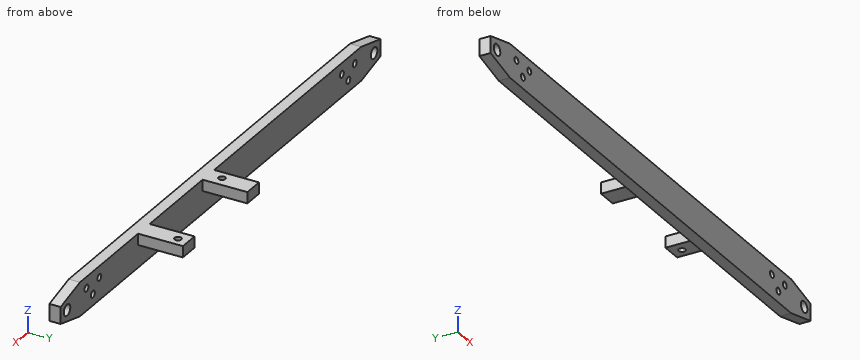
from build123d import *

# Parameters (mm, degrees)
BOSS_EXTRUDE1_DEPTH = 5
SKETCH2_R           = 1.5
SKETCH2_R_2         = 2.5
CUT_EXTRUDE1_DEPTH  = 5
SKETCH4_W           = 9
SKETCH4_H           = 5
BOSS_EXTRUDE2_DEPTH = 20
SKETCH6_R           = 1.5
CUT_EXTRUDE2_DEPTH  = 5


with BuildPart() as part:
    # Sketch1 → Boss-Extrude1 (new body)
    with BuildSketch(Plane(origin=(0, 0, 0), x_dir=(1, 0, 0), z_dir=(0, 1, 0))):
        Polygon((-67.598283163, 7.319100723), (-52.598283163, 3.569100723), (165.401716837, 3.569100723), (180.401716837, 7.319100723), (180.401716837, 14.819100723), (165.401716837, 18.569100723), (-52.598283163, 18.569100723), (-67.598283163, 14.819100723), align=None)
    extrude(amount=BOSS_EXTRUDE1_DEPTH)

    # Sketch2 → Cut-Extrude1 (cut)
    with BuildSketch(Plane(origin=(0, 5, 0), x_dir=(1, 0, 0), z_dir=(0, 1, 0))):
        with Locations(Location((155.401716837, 13.569100723, 0), (0, 0, 270))):
            Circle(SKETCH2_R)
        with Locations(Location((160.401716837, 8.569100723, 0), (0, 0, 270))):
            Circle(SKETCH2_R)
        with Locations(Location((150.401716837, 8.569100723, 0), (0, 0, 270))):
            Circle(SKETCH2_R)
        with Locations(Location((-47.598283163, 8.569100723, 0), (0, 0, 270))):
            Circle(SKETCH2_R)
        with Locations(Location((-37.598283163, 8.569100723, 0), (0, 0, 270))):
            Circle(SKETCH2_R)
        with Locations(Location((-42.598283163, 13.569100723, 0), (0, 0, 270))):
            Circle(SKETCH2_R)
        with Locations(Location((-62.598283163, 11.069100723, 0), (0, 0, 270))):
            Circle(SKETCH2_R_2)
        with Locations(Location((175.401716837, 11.069100723, 0), (0, 0, 270))):
            Circle(SKETCH2_R_2)
    extrude(amount=-CUT_EXTRUDE1_DEPTH, mode=Mode.SUBTRACT)

    # Sketch4 → Boss-Extrude2 (add)
    with BuildSketch(Plane(origin=(-36.696088283, 5, 1.62747237), x_dir=(1, 0, 0), z_dir=(0, 1, 0))):
        with Locations((102.59780512, 7.696573093)):
            Rectangle(SKETCH4_W, SKETCH4_H)
        with Locations((152.59780512, 7.696573093)):
            Rectangle(SKETCH4_W, SKETCH4_H)
    extrude(amount=BOSS_EXTRUDE2_DEPTH)

    # Sketch6 → Cut-Extrude2 (cut)
    with BuildSketch(Plane(origin=(-36.696088283, 0, -3.569100723), x_dir=(1, 0, 0), z_dir=(0, 0, 1))):
        with Locations((102.29780512, 10.9)):
            Circle(SKETCH6_R)
        with Locations((152.89780512, 20.4)):
            Circle(SKETCH6_R)
    extrude(amount=-CUT_EXTRUDE2_DEPTH, mode=Mode.SUBTRACT)


solid = part.part
Source: CAD feature listing. Evaluate the final solid. Frame: model axes, mm. Give positions to 0.01 mm unless a question says otherwise; leave off trailing zeros. Loops run counter-clockwise (first coordinate to the right, second up) from the corner with the lowest first, then second, coordinate; pieces in that order, holes last. Notation, with made-up numbers: (23, -40) -> (33, -40) arc R35 ccw to (33, -3) -> close; hole circle Ø3 at (-20.75, -2.75). An arc over 180 degrees is marked (long way). Use a Markdown table: item, result. Add a question column.
1) Section query A-A, the plane y = 16.25. Return the cut outline in (x, z).
2) First-contact query: pin 1 (8 mm diameter, centred on x = 10.5, z = -16.5, fed in from +Y); pin 2 (8 mm diameter, centred on y = 20, z = -7.5, fed in from -X); pin 3 (10 mm diameter, centred on x = 117, y = 13.5, fed in from -Z); pin 4 (2.5 mm diameter, centred on x = 116.2, y = 20.4, fed in from +Z). Flat tips, straight axial feed; report the tip coordinate or a pass-through.
3) Section query B-B, the plane y = 2. Count the separate pieces of the cut face and the enclosed holes in it, then the cut area to 3 significant figures.
4) Line query: line 1 along X through (y, z) = (5.25, -6.75); line 2 along Y through (x, z) = (76, -8); line 3 along Z through (x, y) = (165.5, 3.5). Output: solid intervals per line, ascending. Write a range as [from, to].
5) Section query C-C, the plane x = 127. Return the cut outline in (y, z).
Numbers:
| question | item | result |
|---|---|---|
| 1 | outline | (61.4, -8.57) -> (70.4, -8.57) -> (70.4, -3.57) -> (61.4, -3.57) -> close; (111.4, -8.57) -> (120.4, -8.57) -> (120.4, -3.57) -> (111.4, -3.57) -> close |
| 2 | pin 1 | stops at y = 5 |
| 2 | pin 2 | stops at x = 61.4 |
| 2 | pin 3 | stops at z = -8.57 |
| 2 | pin 4 | passes through |
| 3 | separate pieces | 1 |
| 3 | enclosed holes | 8 |
| 3 | area | 3,530 mm2 |
| 4 | line 1 | x = [61.4, 70.4], [111.4, 120.4] |
| 4 | line 2 | y = [0, 5] |
| 4 | line 3 | z = [-18.54, -3.59] |
| 5 | outline | (0, -18.57) -> (5, -18.57) -> (5, -3.57) -> (0, -3.57) -> close |
